Part model, mm, in its own coordinate system. A direction names the side the tool comes from. Round coordinates to 2 decimals unless told otherwise and drop trailing zeros. Write each loop counter-clockwise with the first axis right and the second up, starting at its lowest first coordinate (ties: lowest second). Pieces come first, ordered by that corner, then holes. Notation, with made-up numbers: (81, 69.5) -> (123, 69.5) arc R35 cw to (123, 101.5) -> close; hole circle Ø9 at (71, 45.5). An arc over 180 degrees is marked (long way). Use CSV: the item, a comma, the result in double quotes. Start each with the question number.
(1) Saw through at A-A (z = -10.5). Give the cut face in (x, y), plus the area to 4 significant figures.
(2) Two-plate mould, pull along Y, no slides. Class faces 1 (the cylindrical face through (53.531, 14.434, 30.113)), 2 (the cylindrical face through (-26.969, 14.434, 30.113)), 3 (the flat face through (13, 1.5, 20)), 4 (the flat face through (-5, 1, 58.07)): released by +Y, released by -Y, zero draft, split by the parting line, or undercut.
(3) Saw through at B-B (y = 17). Give the cut face in (x, z).
(4) Probe line 1 (X direction, y = 21, z = 15); line 2 (Y direction, x = -10.5, z = 33). List the from-to ranges inside material, lowest first. Write a range as [from, to].
(5) Saw through at C-C (x = 16.5). Give the cut face in (y, z), plus the area to 3 significant figures.
(6) Which spindle directions (+Z, -Z, +X, -X, +Y, -Y) get a long thin tool onto all of the face, cutting with end or side? Do faces 5 (the flat face through (45, 1, -11.93)), 6 (the flat face through (-26.229, 16, 24)), 7 (the flat face through (-19, 1, -11.93)). Say none if no direction does.
(7) Saw through at D-D (z = 12.5). Give the cut face in (x, y), plus the area to 3 significant figures.
(8) Drop flat-ended pins along their axis: pin 1 (0.8 mm diameter, centred on x = -27, y = 16.5, fed in from -Z); pin 2 (8 mm diameter, centred on y = 17, z = 36.3, fed in from +X); pin 3 (0.5 mm diameter, centred on x = -27, y = 28.5, fed in from -Z); pin 4 (1.2 mm diameter, centred on y = 0.5, z = -28, fed in from -X). Give the stop position or say it passes through.
```python
from build123d import *

# Parameters (mm, degrees)
SKETCH1_W           = 82
SKETCH1_H           = 70
BOSS_EXTRUDE1_DEPTH = 1.5
SKETCH2_W           = 1.5
SKETCH2_H           = 70
BOSS_EXTRUDE2_DEPTH = 30
SKETCH3_W           = 11.5
SKETCH3_H           = 12.5
CUT_EXTRUDE1_DEPTH  = 90
SKETCH4_R           = 6.7
CUT_EXTRUDE2_DEPTH  = 90
SKETCH5_W           = 31
SKETCH5_H           = 25
SKETCH5_R           = 6
BOSS_EXTRUDE3_DEPTH = 1.5


with BuildPart() as part:
    # Sketch1 → Boss-Extrude1 (new body)
    with BuildSketch(Plane(origin=(0, 0, 0), x_dir=(1, 0, 0), z_dir=(0, 1, 0))):
        with Locations((13.270768006, -23.069981584)):
            Rectangle(SKETCH1_W, SKETCH1_H)
    extrude(amount=BOSS_EXTRUDE1_DEPTH)

    # Sketch2 → Boss-Extrude2 (add)
    with BuildSketch(Plane(origin=(0, 1.5, 0), x_dir=(1, 0, 0), z_dir=(0, 1, 0))):
        with Locations((53.520768006, -23.069981584)):
            Rectangle(SKETCH2_W, SKETCH2_H)
        with Locations((-26.979231994, -23.069981584)):
            Rectangle(SKETCH2_W, SKETCH2_H)
    extrude(amount=BOSS_EXTRUDE2_DEPTH)

    # Sketch3 → Cut-Extrude1 (cut)
    with BuildSketch(Plane(origin=(54.270768006, 0, 0), x_dir=(0, 0, -1), z_dir=(1, 0, 0))):
        with Locations((6.180018416, 16.95)):
            Rectangle(SKETCH3_W, SKETCH3_H)
    extrude(amount=-CUT_EXTRUDE1_DEPTH, mode=Mode.SUBTRACT)

    # Sketch4 → Cut-Extrude2 (cut)
    with BuildSketch(Plane(origin=(54.270768006, 0, 0), x_dir=(0, 0, -1), z_dir=(1, 0, 0))):
        with Locations((-36.301843463, 17)):
            Circle(SKETCH4_R)
    extrude(amount=-CUT_EXTRUDE2_DEPTH, mode=Mode.SUBTRACT)

    # Sketch5 → Boss-Extrude3 (add)
    with BuildSketch(Plane(origin=(0, 1.5, 0), x_dir=(1, 0, 0), z_dir=(0, 1, 0))):
        with Locations((13.270768006, 24.430018416)):
            Rectangle(SKETCH5_W, SKETCH5_H)
        with Locations(Location((13.270768006, 24.430018416, 0), (0, 0, 270))):
            Circle(SKETCH5_R, mode=Mode.SUBTRACT)
    extrude(amount=-BOSS_EXTRUDE3_DEPTH)


solid = part.part
```
Answers:
1,outline,"(-27.73, 0) -> (54.27, 0) -> (54.27, 10.7) -> (52.77, 10.7) -> (52.77, 1.5) -> (-26.23, 1.5) -> (-26.23, 10.7) -> (-27.73, 10.7) -> close; (-27.73, 23.2) -> (-26.23, 23.2) -> (-26.23, 31.5) -> (-27.73, 31.5) -> close; (52.77, 23.2) -> (54.27, 23.2) -> (54.27, 31.5) -> (52.77, 31.5) -> close"
1,area,"175.5 mm²"
2,face 1,"undercut"
2,face 2,"undercut"
2,face 3,"released by +Y"
2,face 4,"zero draft"
3,outline,"(-27.73, -0.43) -> (-26.23, -0.43) -> (-26.23, 29.6) -> (-27.73, 29.6) -> close; (-27.73, 43) -> (-26.23, 43) -> (-26.23, 58.07) -> (-27.73, 58.07) -> close; (52.77, -0.43) -> (54.27, -0.43) -> (54.27, 29.6) -> (52.77, 29.6) -> close; (52.77, 43) -> (54.27, 43) -> (54.27, 58.07) -> (52.77, 58.07) -> close"
4,line 1,"x = [-27.73, -26.23], [52.77, 54.27]"
4,line 2,"y = [0, 1.5]"
5,outline,"(0, -36.93) -> (1.5, -36.93) -> (1.5, -29.49) -> (0, -29.49) -> close; (0, -19.37) -> (1.5, -19.37) -> (1.5, 58.07) -> (0, 58.07) -> close"
5,area,"127 mm²"
6,face 5,"-Z, +X, +Y, -Y"
6,face 6,"+Z, -Z, +Y"
6,face 7,"-Z, -X, +Y, -Y"
7,outline,"(-27.73, 0) -> (54.27, 0) -> (54.27, 31.5) -> (52.77, 31.5) -> (52.77, 1.5) -> (-26.23, 1.5) -> (-26.23, 31.5) -> (-27.73, 31.5) -> close"
7,area,"213 mm²"
8,pin 1,"stops at z = -0.43"
8,pin 2,"passes through"
8,pin 3,"stops at z = -11.93"
8,pin 4,"stops at x = -2.23"
